Job drawing, mm, ordinate dimensions from the low corner. One solid piece. Round coordinates to 2 decimals unless told otherwise and drop trailing zeros. Loops run counter-clockwise (first coordinate to the right, second up) from the corner with the lowest first, then second, coordinate; pieces in that order, holes last. Notation, with made-up numbers: M 14.25,81 L 19.25,81 A6 cw 19.25,89 Z; hole C 75.5,1 d9. An arc over 180 degrees is marked long. Use one line per item in the form item = value.
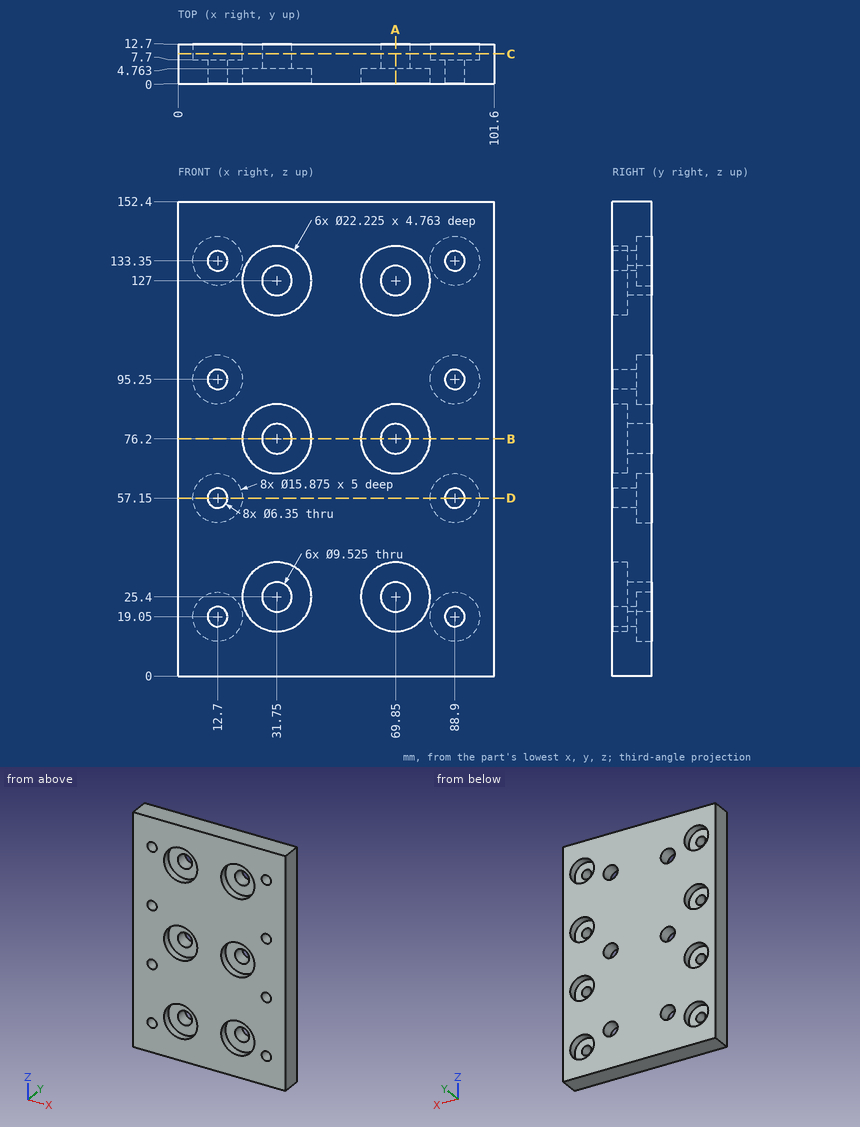
1. Drop flat-ended pins along their axis: P1, Ø6.5, axis at x = 27, z = 126, coming from the -Y side; P2, Ø5, axis at x = 88.9, z = 133.35, coming from the +Y side; P3, Ø8, axis at x = 89.5, z = 98, coming from the +Y side. Give the stop position or say it passes through.
Completed:
P1 = 4.76
P2 = through
P3 = 7.7
2. Cut at D-D on z = 57.15. Write the cut outline in (x, y) (1 decimal), and give its area (3 significant figures).
Completed:
outline = M 0,0 L 9.5,0 L 9.5,7.7 L 4.8,7.7 L 4.8,12.7 L 0,12.7 Z; M 15.9,0 L 85.7,0 L 85.7,7.7 L 81,7.7 L 81,12.7 L 20.6,12.7 L 20.6,7.7 L 15.9,7.7 Z; M 92.1,0 L 101.6,0 L 101.6,12.7 L 96.8,12.7 L 96.8,7.7 L 92.1,7.7 Z
area = 1,030 mm2
3. Cut at B-B on z = 76.2. Write the cut outline in (x, y).
Completed:
outline = M 0,0 L 20.64,0 L 20.64,4.76 L 26.99,4.76 L 26.99,12.7 L 0,12.7 Z; M 36.51,4.76 L 42.86,4.76 L 42.86,0 L 58.74,0 L 58.74,4.76 L 65.09,4.76 L 65.09,12.7 L 36.51,12.7 Z; M 74.61,4.76 L 80.96,4.76 L 80.96,0 L 101.6,0 L 101.6,12.7 L 74.61,12.7 Z
4. Cut at A-A on x = 69.85. Write the cut outline in (y, z), and give its area (3 significant figures).
Completed:
outline = M 0,0 L 12.7,0 L 12.7,20.64 L 4.76,20.64 L 4.76,14.29 L 0,14.29 Z; M 0,36.51 L 4.76,36.51 L 4.76,30.16 L 12.7,30.16 L 12.7,71.44 L 4.76,71.44 L 4.76,65.09 L 0,65.09 Z; M 0,87.31 L 4.76,87.31 L 4.76,80.96 L 12.7,80.96 L 12.7,122.24 L 4.76,122.24 L 4.76,115.89 L 0,115.89 Z; M 0,138.11 L 4.76,138.11 L 4.76,131.76 L 12.7,131.76 L 12.7,152.4 L 0,152.4 Z
area = 1,390 mm2
5. Cut at C-C on y = 9.5. State how many separate pieces and enclosed holes the cut face has, and give its area (3 significant figures).
Completed:
separate_pieces = 1
enclosed_holes = 14
area = 13,500 mm2
6. Probe line 1 along Z through (x, y) = (12.7, 11.55); line 2 along Z through (x, y) = (73, 3.25); line 3 along Z through (x, y) = (12.7, 5.25) (1 decimal). List the from-to ranges inside material, lowest first. Write a range as from..to.
Completed:
line_1 = 0..11.11, 26.99..49.21, 65.09..87.31, 103.19..125.41, 141.29..152.4
line_2 = 0..14.74, 36.06..65.54, 86.86..116.34, 137.66..152.4
line_3 = 0..15.9, 22.2..54, 60.3..92.1, 98.4..130.2, 136.5..152.4
